Source: CAD feature listing. Evaluate the final solid. Frame: model axes, mm. Face numbers are marked on the shaded views. A direction names the side the tool comes from. Give positions to 0.01 mm unless a question says otherwise; leave off trailing zeros. Loops run counter-clockwise (first coordinate to the right, second up) from the corner with the lowest first, then second, coordinate; pieces in that order, holes last. Notation, with made-up numbers: (38, 70.5) -> (96, 70.5) arc R5 cw to (96, 76.5) -> close; hole circle Ø10 at (88.25, 28). An arc over 180 degrees is marked (long way). Put each result on its own line as item: value.
```python
from build123d import *

# Parameters (mm, degrees)
F1_DEPTH = 381
F2_R     = 6.35
F3_DEPTH = 50.801
F5_D     = 8.4328


with BuildPart() as f1:
    # F0 (on Right) → F1 (new body, symmetric)
    with BuildSketch(Plane.YZ):
        Polygon((0, 50.8), (0, 0), (50.8, 0), (50.8, 6.35), (6.35, 6.35), (6.35, 50.8), align=None)
    extrude(amount=F1_DEPTH, both=True)

    # F2 (on face) → F3 (cut, through all)
    with BuildSketch(Plane(origin=(0, 0, 0), x_dir=(1, 0, 0), z_dir=(0, 0, -1))):
        with Locations((0, -25.4)):
            Circle(F2_R)
    extrude(amount=-F3_DEPTH, mode=Mode.SUBTRACT)

    # F5 (through all)
    with Locations(Plane(origin=(0, 0, 0), x_dir=(1, 0, 0), z_dir=(0, 0, -1))):
        with Locations((50.8, -25.4), (-50.8, -25.4)):
            Hole(F5_D / 2)


solid = f1.part
```
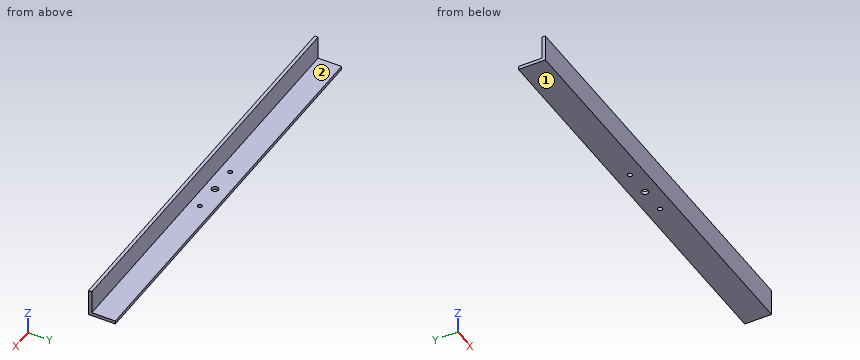
(1) Reachability of the marked faces 1 and 2 from +Z, -Z, +X, -X, +Y, -Y: full face, straight path, thin tool, end or side. Return the list, or none.
Calculated:
face 1: -Z, +X, -X, +Y, -Y
face 2: +Z, +X, -X, +Y
(2) Line query: probe 1 along X at (y, z) = (25, 3); probe 2 along Y at (x, z) = (-50.8, 3); probe 3 along Y at (x, z) = (50, 2). Output: solid intervals per line, ascending. Write a range as from..to.
Calculated:
probe 1: x = -381..-55, -46.6..-6.34, 6.34..46.6, 55..381
probe 2: y = 0..21.18, 29.62..50.8
probe 3: y = 0..21.26, 29.54..50.8
(3) Section C-C on x = -215. Return loops of the section in (y, z).
Calculated:
outline: (0, 0) -> (50.8, 0) -> (50.8, 6.35) -> (6.35, 6.35) -> (6.35, 50.8) -> (0, 50.8) -> close
(4) First-contact query: P1, Ø13.5, axis at x = 120, z = 28, coming from the +Y side; P2, Ø5, axis at x = 50.8, y = 25.4, coming from the -Z side; P3, Ø2, axis at x = -50, y = 13.5, coming from the +Z side; P4, Ø22, axis at x = -60.5, y = 21.5, coming from the +Z side. Flat tips, straight axial feed; report the tip coordinate or a pass-through.
Calculated:
P1: stops at y = 6.35
P2: passes through
P3: stops at z = 6.35
P4: stops at z = 6.35
(5) Section B-B on z = 31.5. Return loops of the section in (x, y), then the cut area to 3 significant figures.
Calculated:
outline: (-381, 0) -> (381, 0) -> (381, 6.35) -> (-381, 6.35) -> close
area: 4,840 mm²
(6) Section A-A on x = 0. Return loops of the section in (y, z), then the cut area to 3 significant figures.
Calculated:
outline: (0, 0) -> (19.05, 0) -> (19.05, 6.35) -> (6.35, 6.35) -> (6.35, 50.8) -> (0, 50.8) -> close; (31.75, 0) -> (50.8, 0) -> (50.8, 6.35) -> (31.75, 6.35) -> close
area: 524 mm²
